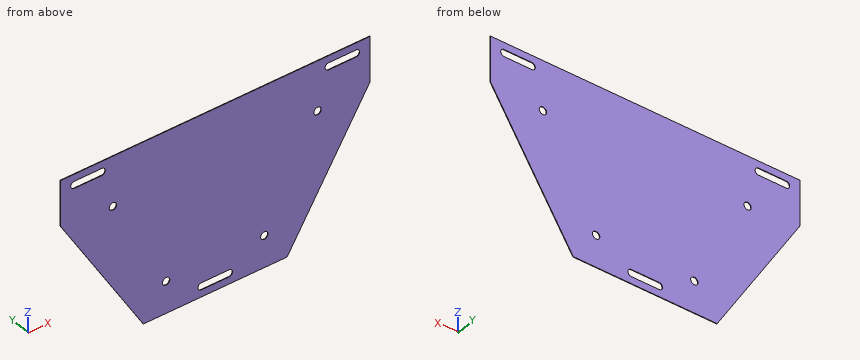
from build123d import *

# Parameters (mm, degrees)
BOSS_EXTRUDE1_DEPTH = 2.65684
CUT_EXTRUDE1_DEPTH  = 1081.026082462
SKETCH3_R           = 16.891
CUT_EXTRUDE2_DEPTH  = 1081.026082462


with BuildPart() as part:
    # Sketch1 → Boss-Extrude1 (new body)
    with BuildSketch(Plane(origin=(0, 0, 0), x_dir=(1, 0, 0), z_dir=(0, 1, 0))):
        Polygon((-711.2, 203.2), (-711.2, 0), (0, 0), (0, 812.8), (-330.2, 812.8), align=None)
        Polygon((0, 812.8), (0, 0), (711.2, 0), (711.2, 203.2), (330.2, 812.8), align=None)
    extrude(amount=BOSS_EXTRUDE1_DEPTH)

    # Sketch2 → Cut-Extrude1 (cut, through all)
    with BuildSketch(Plane(origin=(0, 2.65684, 0), x_dir=(1, 0, 0), z_dir=(0, 1, 0))):
        with BuildLine():
            Line((-63.5, 781.05), (63.5, 781.05))
            ThreePointArc((63.5, 781.05), (79.375, 765.175), (63.5, 749.3))
            Line((63.5, 749.3), (-63.5, 749.3))
            ThreePointArc((-63.5, 749.3), (-79.375, 765.175), (-63.5, 781.05))
        make_face()
        with BuildLine():
            Line((-647.7, 63.5), (-520.7, 63.5))
            ThreePointArc((-520.7, 63.5), (-504.825, 47.625), (-520.7, 31.75))
            Line((-520.7, 31.75), (-647.7, 31.75))
            ThreePointArc((-647.7, 31.75), (-663.575, 47.625), (-647.7, 63.5))
        make_face()
        with BuildLine():
            Line((520.7, 63.5), (647.7, 63.5))
            ThreePointArc((647.7, 63.5), (663.575, 47.625), (647.7, 31.75))
            Line((647.7, 31.75), (520.7, 31.75))
            ThreePointArc((520.7, 31.75), (504.825, 47.625), (520.7, 63.5))
        make_face()
    extrude(amount=-CUT_EXTRUDE1_DEPTH, mode=Mode.SUBTRACT)

    # Sketch3 → Cut-Extrude2 (cut, through all)
    with BuildSketch(Plane(origin=(0, 2.65684, 0), x_dir=(1, 0, 0), z_dir=(0, 1, 0))):
        with Locations(Location((-469.9, 224.282, 0), (0, 0, 270))):
            Circle(SKETCH3_R)
        with Locations(Location((-225.425, 669.586361505, 0), (0, 0, 270))):
            Circle(SKETCH3_R)
        with Locations(Location((225.425, 669.586361505, 0), (0, 0, 270))):
            Circle(SKETCH3_R)
        with Locations(Location((469.9, 224.282, 0), (0, 0, 270))):
            Circle(SKETCH3_R)
    extrude(amount=-CUT_EXTRUDE2_DEPTH, mode=Mode.SUBTRACT)


solid = part.part
Work out the finished part from the listing and answer in its coordinate system (mm). Round coordinates to 2 decimals unless told otherwise and drop trailing zeros. Write each loop counter-clockwise with the first axis right and the second up, starting at its lowest first coordinate (ties: lowest second). Pieces come first, ordered by that corner, then holes. Notation, with made-up numbers: (-12.5, 73.5) - (16.5, 73.5) arc R14 cw to (16.5, 86.5) - close; hole circle Ø4 at (-29.75, -35). An arc over 180 degrees is marked (long way). Answer in a Markdown table with one row per item. Add a question column.
1. A cutting plane is placed at C-C, the plane z = -269. Determine the outline of the cut face in (x, y) (3 decimals), and give its area (3 significant figures).
2. Given pin 1 (1 mm diameter, centred on x = -190, z = -708, fed in from -Y); pin 2 (0.8 mm diameter, centred on x = 612.5, y = 1, fed in from -Z); pin 3 (0.8 mm diameter, centred on x = -575, y = 1, fed in from -Z), each flat-ended and moving along its own axis, determine where each tip first touches the part or whether it passes through.
3. A cutting plane is placed at B-B, the plane y = 0.85. Determine the outline of the cut face in (x, z) (3 decimals), and give its area (3 significant figures).
4. Find the intervals of material crossed by line 1 along Z through (x, y) = (-31.5, 1.2); line 2 along X through (y, z) = (0.4, -774); line 3 along Z through (x, y) = (651, 1.3), in increasing order. Write a range as from..to.
5. A cutting plane is placed at A-A, the plane x = 469.9. Determine the outline of the cut face in (y, z), and give its area (3 significant figures).
6. A cutting plane is placed at D-D, the plane z = -734.5. Determine the outline of the cut face in (x, y), and give its area (3 significant figures).
Worked out:
| question | item | result |
|---|---|---|
| 1 | outline | (-670.075, 0) - (670.075, 0) - (670.075, 2.657) - (-670.075, 2.657) - close |
| 1 | area | 3,560 mm^2 |
| 2 | pin 1 | y = 0 |
| 2 | pin 2 | z = -361.76 |
| 2 | pin 3 | z = -421.76 |
| 3 | outline | (-711.2, -203.2) - (-330.2, -812.8) - (330.2, -812.8) - (711.2, -203.2) - (711.2, 0) - (-711.2, 0) - close; hole (-647.7, -63.5) - (-520.7, -63.5) arc R15.875 ccw to (-520.7, -31.75) - (-647.7, -31.75) arc R15.875 ccw to start; hole circle Ø33.782 at (-469.9, -224.282); hole circle Ø33.782 at (-225.425, -669.586); hole (-63.5, -781.05) - (63.5, -781.05) arc R15.875 ccw to (63.5, -749.3) - (-63.5, -749.3) arc R15.875 ccw to start; hole circle Ø33.782 at (225.425, -669.586); hole circle Ø33.782 at (469.9, -224.282); hole (520.7, -63.5) - (647.7, -63.5) arc R15.875 ccw to (647.7, -31.75) - (520.7, -31.75) arc R15.875 ccw to start |
| 3 | area | 906,000 mm^2 |
| 4 | line 1 | -812.8..-781.05, -749.3..0 |
| 4 | line 2 | -354.45..-76.7, 76.7..354.45 |
| 4 | line 3 | -299.52..-63.15, -32.1..0 |
| 5 | outline | (0, -589.28) - (2.66, -589.28) - (2.66, -241.17) - (0, -241.17) - close; (0, -207.39) - (2.66, -207.39) - (2.66, 0) - (0, 0) - close |
| 5 | area | 1,480 mm^2 |
| 6 | outline | (-379.14, 0) - (379.14, 0) - (379.14, 2.66) - (-379.14, 2.66) - close |
| 6 | area | 2,010 mm^2 |
